Read the model definition and answer for the solid it produces. Units are mm, in the model's axes. A direction names the side the tool comes from. Give positions to 0.01 mm unless a question says otherwise; leave off trailing zeros. Write each loop counter-clockwise with the first axis right and the second up, starting at its lowest first coordinate (ties: lowest second). Pieces come first, ordered by that corner, then holes.
```python
from build123d import *

# Parameters (mm, degrees)
SKETCH1_W           = 127
SKETCH1_H           = 50.8
BOSS_EXTRUDE1_DEPTH = 50.8
SKETCH2_W           = 18.996127276
SKETCH2_H           = 50.8
SKETCH2_W_2         = 19.127407137
CUT_EXTRUDE1_DEPTH  = 44.45
SKETCH3_W           = 76.151334044
SKETCH3_H           = 50.8
CUT_EXTRUDE2_DEPTH  = 44.45
SKETCH5_R           = 3.937
CUT_EXTRUDE4_DEPTH  = 44.45
SKETCH6_R           = 3.937
CUT_EXTRUDE5_DEPTH  = 44.45


with BuildPart() as part:
    # Sketch1 → Boss-Extrude1 (new body)
    with BuildSketch(Plane.XY):
        Rectangle(SKETCH1_W, SKETCH1_H)
    extrude(amount=BOSS_EXTRUDE1_DEPTH)

    # Sketch2 → Cut-Extrude1 (cut)
    with BuildSketch(Plane(origin=(0, 0, 0), x_dir=(-1, 0, 0), z_dir=(0, 0, -1))):
        with Locations((-54.001936362, 0)):
            Rectangle(SKETCH2_W, SKETCH2_H)
        with Locations((53.936296432, 0)):
            Rectangle(SKETCH2_W_2, SKETCH2_H)
    extrude(amount=-CUT_EXTRUDE1_DEPTH, mode=Mode.SUBTRACT)

    # Sketch3 → Cut-Extrude2 (cut)
    with BuildSketch(Plane.XY.offset(50.8)):
        Rectangle(SKETCH3_W, SKETCH3_H)
    extrude(amount=-CUT_EXTRUDE2_DEPTH, mode=Mode.SUBTRACT)

    # Sketch5 → Cut-Extrude4 (cut)
    with BuildSketch(Plane(origin=(0, 0, 44.45), x_dir=(-1, 0, 0), z_dir=(0, 0, -1))):
        with Locations((-54.001936362, 0)):
            Circle(SKETCH5_R)
    extrude(amount=-CUT_EXTRUDE4_DEPTH, mode=Mode.SUBTRACT)

    # Sketch6 → Cut-Extrude5 (cut)
    with BuildSketch(Plane(origin=(0, 0, 44.45), x_dir=(-1, 0, 0), z_dir=(0, 0, -1))):
        with Locations((53.936296432, 0)):
            Circle(SKETCH6_R)
    extrude(amount=-CUT_EXTRUDE5_DEPTH, mode=Mode.SUBTRACT)


solid = part.part
```
Item 1: Section C-C (z = 31.5) is taken. Write down the section's boundary in (x, y), and give its area (3 significant figures).
Result set:
outline: (-44.37, -25.4) - (-38.08, -25.4) - (-38.08, 25.4) - (-44.37, 25.4) - close; (38.08, -25.4) - (44.5, -25.4) - (44.5, 25.4) - (38.08, 25.4) - close
area: 646 mm2
Item 2: Section A-A (y = 0) is taken. Write down the section's boundary in (x, z).
Result set:
outline: (-63.5, 44.45) - (-57.87, 44.45) - (-57.87, 50.8) - (-63.5, 50.8) - close; (-50, 44.45) - (-44.37, 44.45) - (-44.37, 0) - (44.5, 0) - (44.5, 44.45) - (50.06, 44.45) - (50.06, 50.8) - (38.08, 50.8) - (38.08, 6.35) - (-38.08, 6.35) - (-38.08, 50.8) - (-50, 50.8) - close; (57.94, 44.45) - (63.5, 44.45) - (63.5, 50.8) - (57.94, 50.8) - close
Item 3: Find the intervals of material crossed by line 1 along X through (y, z) = (1, 9.5); line 2 along Z through (x, y) = (-30, -7); line 3 along Z through (x, y) = (-57, -16.5), in increasing order.
Result set:
line 1: x = -44.37 to -38.08, 38.08 to 44.5
line 2: z = 0 to 6.35
line 3: z = 44.45 to 50.8
Item 4: Determine the mould class of faces 1 (the flat face through (0, -25.4, 5)), 2 (the cylindrical face through (57.935, 0.173, 47.581)), 3 (the cylindrical face through (-57.691, 1.183, 47.581)), 4 (the flat face through (-48, 0, 50.8)) for opening direction Y: pulls with the +Y half, pulls with the -Y half, needs draft (parallel to the pull), parting line crosses it, or undercut.
Result set:
face 1: pulls with the -Y half
face 2: undercut
face 3: undercut
face 4: needs draft
Item 5: Each of these flat-tipped pins is pushed along its axis until it touches: pin 1 Ø22 at (y, z) = (10, 29.5) entering from +X; pin 2 Ø12.5 at (x, y) = (54, 0) entering from +Z; pin 3 Ø1 at (y, z) = (7.5, 11.5) entering from -X; pin 4 Ø15 at (x, y) = (56, 5) entering from -Z. Where does it stop, or does it pass through?
Result set:
pin 1: stops at x = 44.5
pin 2: stops at z = 50.8
pin 3: stops at x = -44.37
pin 4: stops at z = 44.45
Item 6: Which of the six approach directions +Z, -Z, +X, -X, +Y, -Y give full straight-line access (tool end or side, diameter ignored) to faces 5 (the flat face through (58.4, 0.4, 44.45)), 6 (the flat face through (63.5, 0, 48)), 7 (the flat face through (-49.6, 0.4, 44.45)), 8 (the flat face through (-1, 0, 6.35))?
Result set:
face 5: -Z, +X, +Y, -Y
face 6: +Z, -Z, +X, +Y, -Y
face 7: -Z, -X, +Y, -Y
face 8: +Z, +Y, -Y
Item 7: Section D-D (y = 14) is taken. Write down the section's boundary in (x, z), and give its area (3 significant figures).
Result set:
outline: (-63.5, 44.45) - (-44.37, 44.45) - (-44.37, 0) - (44.5, 0) - (44.5, 44.45) - (63.5, 44.45) - (63.5, 50.8) - (38.08, 50.8) - (38.08, 6.35) - (-38.08, 6.35) - (-38.08, 50.8) - (-63.5, 50.8) - close
area: 1,370 mm2
Item 8: Section B-B (z = 46.5) is taken. Write down the section's boundary in (x, y).
Result set:
outline: (-63.5, -25.4) - (-38.08, -25.4) - (-38.08, 25.4) - (-63.5, 25.4) - close; (38.08, -25.4) - (63.5, -25.4) - (63.5, 25.4) - (38.08, 25.4) - close; hole circle Ø7.87 at (-53.94, 0); hole circle Ø7.87 at (54, 0)
